```python
from build123d import *

# Parameters (mm, degrees)
F1_DEPTH    = 2
F2_T1_DEPTH = 2


# Not quite as in the source:
# - a fillet or chamfer that OpenCascade refuses, or shapes differently, is made with other operations: its cross-section is extruded or revolved along the edge and cut away or added


with BuildPart() as f1:
    # F0 (on Front) → F1 (new body)
    with BuildSketch(Plane.XZ):
        with BuildLine():
            Line((-11.6313876303, 13), (-11.6313876303, 0))
            Line((-11.6313876303, 0), (-8.150026169, 0))
            Line((-8.150026169, 0), (-7.9982068951, -7.1693707857))
            ThreePointArc((-7.9982068951, -7.1693707857), (0.1698610087, -14.9981964991), (7.998186073, -6.829648769))
            Line((7.998186073, -6.829648769), (7.998186073, 0))
            Line((7.998186073, 0), (11.8686123697, 0))
            Line((11.8686123697, 0), (11.8686123697, 13))
            ThreePointArc((11.8686123697, 13), (0.1186123697, 21), (-11.6313876303, 13))
        make_face()
        with BuildLine():
            ThreePointArc((-4.9980202119, -7.1406910146), (-5, -7), (-4.9980202119, -6.8593089854))
            Line((-4.9980202119, -6.8593089854), (-4.9980202119, 1.395497035))
            ThreePointArc((-4.9980202119, 1.395497035), (0.2650718597, 17.7983630087), (4.9915903324, 1.2329118096))
            Line((4.9915903324, 1.2329118096), (4.9915903324, -6.7101276944))
            ThreePointArc((4.9915903324, -6.7101276944), (0.2153056642, -11.9953621962), (-4.9980202119, -7.1406910146))
        make_face(mode=Mode.SUBTRACT)
    extrude(amount=F1_DEPTH)

    # F2: fillet of radius 6.5 on 2 edges, made by hand

    # F2_s2 → F2_t1 (join)
    with BuildSketch(Plane.XZ):
        with BuildLine():
            ThreePointArc((-11.6313876303, 0), (-9.0385133393, -2.3384510594), (-8.029721431, -5.6811579463))
            Line((-8.029721431, -5.6811579463), (-8.150026169, 0))
            Line((-8.150026169, 0), (-11.6313876303, 0))
        make_face()
        with BuildLine():
            ThreePointArc((7.998186073, -5.9443538033), (9.0510662344, -2.3976813538), (11.8686123697, 0))
            Line((11.8686123697, 0), (7.998186073, 0))
            Line((7.998186073, 0), (7.998186073, -5.9443538033))
        make_face()
    extrude(amount=F2_T1_DEPTH)


solid = f1.part
```
Check sheet for the modelled part. Datum: model origin and axes. Units: mm. A direction names the side the tool comes from. Round coordinates to 2 decimals unless told otherwise and drop trailing zeros. Order: outer loops, then holes, each group sorted by start corner. A loop starts at its lowest first (then second) coordinate and runs counter-clockwise, first axis right, second up. Notation, with made-up numbers: (11, 14.5) -> (44, 14.5) arc R32 ccw to (44, 45.5) -> close; hole circle Ø8 at (10, 11). An arc over 180 degrees is marked (long way). One line per item, written item: value. Start each with the question number.
Q1. Thickness scan on line 1 (X direction, y = -1.1, z = 15); line 2 (Z direction, x = 0.75, y = -1.4); line 3 (X direction, y = -1.5, z = -8). Record the ranges inside material, lowest first.
Q2. Mould release check, pull along Z, two halves, no side actions. Record for faces 4 (the face through (5.2, -2, -0.7)), 5 (the face through (0, -1, 21)), 6 (the face through (-0.057, -0.986, 17.798)), 7 (the face through (4.992, -1, -3)): pulls with the +Z half, pulls with the -Z half, needs draft (parallel to the pull), parting line crosses it, or undercut.
Q3. Gauge pin test, flat ends, axial feed: pin 1 Ø0.6 at (y, z) = (-1, -4.5) entering from +X; pin 2 Ø5 at (x, z) = (-3.5, 13.5) entering from -Y. Record the tip position at first contact, or that the pin passes through.
Q4. Cross-section at D-D (x = -9.75). Record the boundary of the cut face in (y, z), and give its area (3 significant figures).
Q5. Cross-section at B-B (z = 15.5). Record the boundary of the cut face in (x, y), and give its area (3 significant figures).
Q6. Cross-section at A-A (y = -1.5). Record the boundary of the cut face in (x, z), and give its area (3 significant figures).
Q7. Set-up check for faces 1 (the face through (-4.998, -1, -3)), 2 (the face through (5.2, 0, -0.7)), 3 (the face through (7.998, -1, -6.4)): record each of +Z, -Z, +X, -X, +Y, -Y from which the full face is reachable in a straight line by a thin tool's end or side.
Q8. Cross-section at C-C (x = 8.5). Record the boundary of the cut face in (y, z), and give its area (3 significant figures).
Completed:
1. line 1: x = -10.63 to -6.4, 6.64 to 10.87
1. line 2: z = -14.96 to -11.94, 17.78 to 20.98
1. line 3: x = -7.94 to -4.9, 4.9 to 7.94
2. face 4: needs draft
2. face 5: pulls with the +Z half
2. face 6: undercut
2. face 7: undercut
3. pin 1: stops at x = 8.24
3. pin 2: passes through
4. outline: (-2, -1.41) -> (0, -1.41) -> (0, 16.25) -> (-2, 16.25) -> close
4. area: 35.3 mm²
5. outline: (-10.31, -2) -> (-5.89, -2) -> (-5.89, 0) -> (-10.31, 0) -> close; (6.13, -2) -> (10.54, -2) -> (10.54, 0) -> (6.13, 0) -> close
5. area: 17.7 mm²
6. outline: (-11.63, 0) arc R6.5 cw to (-8.03, -5.68) -> (-8, -7.17) arc R8 ccw to (8, -6.83) -> (8, -5.94) arc R6.5 cw to (11.87, 0) -> (11.87, 13) arc R12.63 ccw to (-11.63, 13) -> close; hole (-5, -6.86) arc R5 ccw (long way) to (4.99, -6.71) -> (4.99, 1.23) arc R9 ccw (long way) to (-5, 1.4) -> close
6. area: 300 mm²
7. face 1: +Y, -Y
7. face 2: +Z, -Z, +X, -X, +Y
7. face 3: -Z, +X, +Y, -Y
8. outline: (-2, -3.44) -> (0, -3.44) -> (0, 5.52) -> (-2, 5.52) -> close; (-2, 12.08) -> (0, 12.08) -> (0, 17.82) -> (-2, 17.82) -> close
8. area: 29.4 mm²
